Could you check a few things on this model? Use its own coordinates, in mm. A direction names the side the tool comes from. Round coordinates to 2 decimals unless told otherwise and drop trailing zeros. Loops run counter-clockwise (first coordinate to the right, second up) from the corner with the lowest first, then second, coordinate; pieces in that order, holes last. Notation, with made-up numbers: (43.25, -39) -> (65.25, -39) arc R17 cw to (65.25, -19) -> close; hole circle Ø10 at (-3.5, -26.5). An arc over 180 degrees is marked (long way). One line per item, written item: value.
Autodesk Inventor part; units mm, degrees
ref_plane "YZ Plane" through (0, 0, 0) normal (1, 0, 0) x (0, 1, 0)
ref_plane "XZ Plane" through (0, 0, 0) normal (0, 1, 0) x (-1, 0, 0)
ref_plane "XY Plane" through (0, 0, 0) normal (0, 0, 1) x (1, 0, 0)
sketch "Sketch1" plane through (0, 0, 0) normal (0, 0, 1) x (1, 0, 0)
  line L0 (0, 0) -> (0, 10) construction
  line L1 (0, 31.5) -> (10, 31.5)
  line L2 (10, 31.5) -> (10, 27)
  line L3 (10, 27) -> (15, 27)
  line L4 (15, 27) -> (15, 47.5)
  line L5 (15, 47.5) -> (28, 47.5)
  line L6 (28, 47.5) -> (28, 14)
  line L7 (28, 0) -> (0, 0)
  line L8 (0, 10) -> (24, 10)
  line L9 (24, 10) -> (24, 14)
  line L10 (24, 14) -> (28, 14)
  line L11 (0, 10) -> (0, 31.5)
  line L12 (28, 14) -> (28, 0) construction
  dimension "d0" = 95
  dimension "d1" = 54
  dimension "d2" = 63
  dimension "d3" = 20
  dimension "d4" = 28
  dimension "d5" = 4
  dimension "d6" = 28
  dimension "d7" = 13
  dimension "d8" = 10
revolve "Revolution1" add sketch "Sketch1" angle 360 about axis through (28, 0, 0) along (-1, 0, 0)
chamfer "Chamfer1" distance 1 angle 45 4 edges at (24, -10, 0) (0, -10, 0) (10, -31.5, 0) (0, -31.5, 0)
sketch "Sketch2" plane through (28, 0, 0) normal (1, 0, 0) x (0, 0, -1)
  circle A0 centre (0, 0) radius 47.5
  circle A1 centre (0, 0) radius 14
  arc A2 (3.2661, -26.6002) -> (25.02, -9.6043) centre (0, 0) ccw
  arc A3 (2.8883, -23.5233) -> (22.1259, -8.4933) centre (0, 0) ccw
  line L0 (2.8883, -23.5233) -> (3.2661, -26.6002)
  line L1 (22.1259, -8.4933) -> (25.02, -9.6043)
  line L2 (0, 0) -> (0, -47.5)
  dimension "d13" = 7
  dimension "d14" = 62
  dimension "d15" = 23.7
  dimension "d16" = 26.8
extrude "Extrusion1" add sketch "Sketch2" along normal blind 10 contours L0 A3 L1 A2
sketch "Sketch3" plane through (28, 0, 0) normal (1, 0, 0) x (0, 0, -1)
  arc A0 (2.8883, -23.5233) -> (22.1259, -8.4933) centre (0, 0) ccw
  circle A1 centre (0, 0) radius 47.5
  line L0 (-34.165, 33) -> (-15, 33)
  line L1 (-15, 33) -> (-15, 45.0694)
  dimension "d19" = 33
  dimension "d20" = 15
extrude "Extrusion2" cut sketch "Sketch3" against normal through all contours L1 L0 A1 picked at (-25.8726, 34.6785)
sketch "Sketch4" plane through (28, 33, 15) normal (1, 0, 0) x (0, 0, -1)
  circle A0 centre (15, -33) radius 14
  line L0 (0, 0) -> (-19.165, 0)
  point P0 (15, 6)
  dimension "d23" = 6
hole "Hole1" at (28, 39, 0) direction (-1, 0, 0) diameter 10 end through all
sketch "Sketch5" plane through (28, 33, 15) normal (0, 0, 1) x (1, 0, 0)
  line L0 (0, 0) -> (-13, 0)
  line L1 (-13, 12.0694) -> (0, 12.0694)
  point P0 (-28, -33)
  point P1 (-6.5, 6)
  point P2 (-6.5, 12.0694)
  dimension "d31" = 6
hole "Hole2" at (21.5, 39, 15) direction (0, 0, -1) diameter 4.917 end up to surface
pattern_circular "Circular Pattern1" count 2 over 120 about axis through (21.5, 0, 0) along (1, 0, 0) of "Hole2", "Hole1", "Extrusion2"
sketch "Sketch6" plane through (24, 0, 0) normal (1, 0, 0) x (0, 0, -1)
  circle A0 centre (0, 0) radius 14
  line L0 (-3, 0) -> (3, 0)
  line L1 (3, 0) -> (3, 12.3)
  line L2 (3, 12.3) -> (-3, 12.3)
  line L3 (-3, 12.3) -> (-3, 0)
  dimension "d42" = 12.3
  dimension "d43" = 6
extrude "Extrusion3" cut sketch "Sketch6" against normal through all contours L3 L2 L1 L0
properties part number "Part032.Front support" material "Steel, Cast"
(1) If we section it at B-B, the plane x = 5.5: Please give me the cut outline in (y, z), then the cut area to 3 significant figures.
Recorded:
outline: circle Ø63 at (0, 0); hole (9.54, -3) -> (12.3, -3) -> (12.3, 3) -> (9.54, 3) arc R10 ccw (long way) to start
area: 2,790 mm²
(2) If we section it at C-C, the plane y = 0: Please give me the cut outline in (x, z), then the cut area to 3 significant figures.
Recorded:
outline: (0, -30.5) -> (1, -31.5) -> (9, -31.5) -> (10, -30.5) -> (10, -27) -> (15, -27) -> (15, -47.5) -> (28, -47.5) -> (28, -14) -> (24, -14) -> (24, -11) -> (23, -10) -> (1, -10) -> (0, -11) -> close; (0, 11) -> (1, 10) -> (23, 10) -> (24, 11) -> (24, 14) -> (28, 14) -> (28, 47.5) -> (15, 47.5) -> (15, 27) -> (10, 27) -> (10, 30.5) -> (9, 31.5) -> (1, 31.5) -> (0, 30.5) -> close
area: 1,540 mm²
(3) If we section it at D-D, the plane y = 39: Please give me the cut outline in (x, z).
Recorded:
outline: (15, -27.12) -> (28, -27.12) -> (28, -5) -> (15, -5) -> close; (15, 5) -> (19.04, 5) -> (19.04, 15) -> (15, 15) -> close; (23.96, 5) -> (28, 5) -> (28, 15) -> (23.96, 15) -> close
(4) For faces 1 (the face through (24, -9.4, -6.3)), 2 (the face through (15, 20, 20)), 3 (the face through (32.93, -18.565, -14.732)), 4 (the face through (22, 33, 25)), which set-ups out of +Z, -Z, +X, -X, +Y, -Y let a thin tool reach every point of the face, with its end or its side?
Recorded:
face 1: +X
face 2: none
face 3: +Z, +X, +Y
face 4: +Z, +X, -X, +Y
(5) If we section it at A-A, the plane z = 0: Give the number of separate pieces and of enclosed holes in the cut face, then the cut area to 3 significant figures.
Recorded:
separate pieces: 3
enclosed holes: 0
area: 1,350 mm²
(6) I'm going to push flat-ended pins straight in: pin 1 Ø16 at (y, z) = (-19.5, 33.77) entering from -X; pin 2 Ø1 at (x, y) = (20.5, -28) entering from +Z; pin 3 Ø12 at (x, y) = (21, -9.5) entering from +Z; pin 4 Ø12 at (y, z) = (0, 0) entering from -X. Where does each tip first touch, or does it pass through?
Recorded:
pin 1: x = 0.5
pin 2: z = 38.73
pin 3: z = 47.37
pin 4: through
(7) If I drill on L1, parallel to Y at x = 26.4, z = 0; L2, parallel to Z at x = 25, y = 0; L3, parallel to X at y = 39, z = 10, over which ranges is the centre line in solid material (lowest first)?
Recorded:
L1: -47.5 to -14, 14 to 34, 44 to 47.5
L2: -47.5 to -14, 14 to 47.5
L3: 15 to 19.04, 23.96 to 28
(8) Thinking about a two-plate mould opening in Z: for faces 5 (the face through (21.41, -14.62, 34.86)), 6 (the face through (22.44, 36.73, 9.6)), 7 (the face through (26.028, 12.932, -5.362)), 8 (the face through (32.93, -25.04, -3.075)), which applies, released by +Z, released by -Z, zero draft, split by the parting line, or undercut?
Recorded:
face 5: undercut
face 6: zero draft
face 7: undercut
face 8: released by +Z
